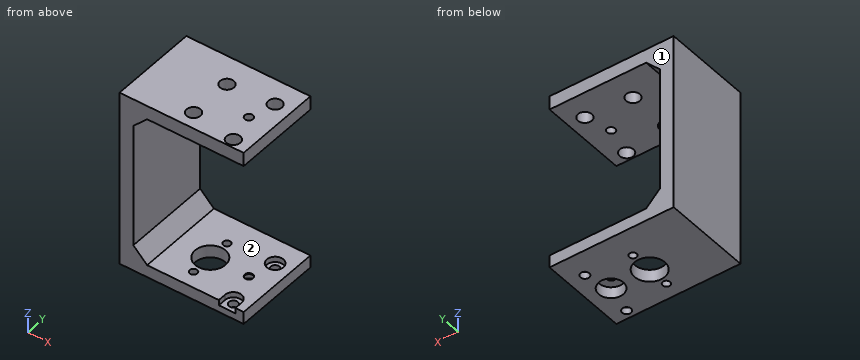
from build123d import *

# Parameters (mm, degrees)
SKETCH1_R           = 5.5
SKETCH1_R_2         = 4.45
BOSS_EXTRUDE1_DEPTH = 4.5
BOSS_EXTRUDE2_START = -0.4
SKETCH2_R           = 4.45
SKETCH2_R_2         = 1.5
BOSS_EXTRUDE2_DEPTH = 0.4
SKETCH3_R           = 1.6
CUT_EXTRUDE1_DEPTH  = 10
SKETCH4_R           = 1.35
CUT_EXTRUDE2_DEPTH  = 10
SKETCH5_W           = 45
SKETCH5_H           = 4.5
BOSS_EXTRUDE3_DEPTH = 4.5
SKETCH6_R           = 3
CUT_EXTRUDE4_DEPTH  = 2
SKETCH7_W           = 5
SKETCH7_H           = 32
BOSS_EXTRUDE4_DEPTH = 60
SKETCH8_W           = 5
SKETCH8_H           = 32
BOSS_EXTRUDE5_DEPTH = 40
CUT_EXTRUDE5_START  = -5
SKETCH11_R          = 2.5
SKETCH11_R_2        = 1.5
CUT_EXTRUDE5_DEPTH  = 5
CHAMFER1_SIZE       = 5


with BuildPart() as part:
    # Sketch1 → Boss-Extrude1 (new body)
    with BuildSketch(Plane.XY):
        Polygon((0, 27.5), (32.5, 27.5), (32.5, 0), (0, 0), (-12.5, 0), (-12.5, 27.5), align=None)
        with Locations((10, 13.75)):
            Circle(SKETCH1_R, mode=Mode.SUBTRACT)
        with Locations((24, 13.75)):
            Circle(SKETCH1_R_2, mode=Mode.SUBTRACT)
    extrude(amount=BOSS_EXTRUDE1_DEPTH)

    # Sketch2 → Boss-Extrude2 (add)
    with BuildSketch(Plane.XY.offset(4.5).offset(BOSS_EXTRUDE2_START)):
        with Locations((24, 13.75)):
            Circle(SKETCH2_R)
        with Locations((24, 13.75)):
            Circle(SKETCH2_R_2, mode=Mode.SUBTRACT)
    extrude(amount=BOSS_EXTRUDE2_DEPTH)

    # Sketch3 → Cut-Extrude1 (cut)
    with BuildSketch(Plane.XY.offset(4.5)):
        with Locations((26.5, 23)):
            Circle(SKETCH3_R)
        with Locations((26.5, 3)):
            Circle(SKETCH3_R)
    extrude(amount=-CUT_EXTRUDE1_DEPTH, mode=Mode.SUBTRACT)

    # Sketch4 → Cut-Extrude2 (cut)
    with BuildSketch(Plane.XY.offset(4.5)):
        with Locations((10, 21.75)):
            Circle(SKETCH4_R)
        with Locations((10, 5.75)):
            Circle(SKETCH4_R)
    extrude(amount=-CUT_EXTRUDE2_DEPTH, mode=Mode.SUBTRACT)

    # Sketch5 → Boss-Extrude3 (add)
    with BuildSketch(Plane.XY.offset(4.5)):
        with Locations((10, 29.75)):
            Rectangle(SKETCH5_W, SKETCH5_H)
    extrude(amount=-BOSS_EXTRUDE3_DEPTH)

    # Sketch6 → Cut-Extrude4 (cut)
    with BuildSketch(Plane.XY.offset(4.5)):
        with Locations((26.5, 23)):
            Circle(SKETCH6_R)
        with BuildLine():
            Line((23.5, 3), (23.5, 0))
            Line((23.5, 0), (29.5, 0))
            Line((29.5, 0), (29.5, 3))
            ThreePointArc((29.5, 3), (26.5, 6), (23.5, 3))
        make_face()
    extrude(amount=-CUT_EXTRUDE4_DEPTH, mode=Mode.SUBTRACT)

    # Sketch7 → Boss-Extrude4 (add)
    with BuildSketch(Plane.XY.offset(4.5)):
        with Locations((-10, 16)):
            Rectangle(SKETCH7_W, SKETCH7_H)
    extrude(amount=BOSS_EXTRUDE4_DEPTH)

    # Sketch8 → Boss-Extrude5 (add)
    with BuildSketch(Plane(origin=(-7.5, 0, 0), x_dir=(0, 0, -1), z_dir=(1, 0, 0))):
        with Locations((-62, 16)):
            Rectangle(SKETCH8_W, SKETCH8_H)
    extrude(amount=BOSS_EXTRUDE5_DEPTH)

    # Sketch11 → Cut-Extrude5 (cut)
    with BuildSketch(Plane.XY.offset(64.5).offset(CUT_EXTRUDE5_START)):
        with Locations((10, 21.75)):
            Circle(SKETCH11_R)
        with Locations((26.5, 23)):
            Circle(SKETCH11_R)
        with Locations((26.5, 3)):
            Circle(SKETCH11_R)
        with Locations((10, 5.75)):
            Circle(SKETCH11_R)
        with Locations((24, 13.75)):
            Circle(SKETCH11_R_2)
    extrude(amount=CUT_EXTRUDE5_DEPTH, mode=Mode.SUBTRACT)

    # Chamfer1
    chamfer1_edges = [part.edges().sort_by_distance(p)[0] for p in [
        (-7.5, 16, 59.5),
        (-7.5, 16, 4.5),
    ]]
    chamfer(chamfer1_edges, length=CHAMFER1_SIZE)


solid = part.part
Part model, mm, in its own coordinate system. Face numbers are marked on the shaded views. A direction names the side the tool comes from. Coordinates: 2 decimals unless noted, no trailing zeros. Order: outer loops, then holes, each group sorted by start corner. A loop starts at its lowest first (then second) coordinate and runs counter-clockwise, first axis right, second up.
(1) Tool access for the marked faces 1 and 2: list every direction of +Z, -Z, +X, -X, +Y, -Y with a clear straight run to the whole face (end or side of a thin tool).
Check sheet entries:
face 1: +Z, -Z, +X, -X, +Y
face 2: +X, +Y, -Y
(2) Probe L1, parallel to Y at x = 10, z = 3.5; L2, parallel to Y at x = 26.5, z = 61.1; L3, parallel to Z at x = 21, y = 25.5. List the from-to ranges inside material, lowest first.
Check sheet entries:
L1: y = 0 to 4.4, 7.1 to 8.25, 19.25 to 20.4, 23.1 to 32
L2: y = 0 to 0.5, 5.5 to 20.5, 25.5 to 32
L3: z = 0 to 4.5, 59.5 to 64.5
(3) Pin check, flat tips, straight feed: pin 1 Ø12 at (y, z) = (27, 32.5) entering from +X; pin 2 Ø1.8 at (x, y) = (27.5, 2.5) entering from +Z. Stop position of each tip, or through.
Check sheet entries:
pin 1: stops at x = -7.5
pin 2: stops at z = 2.5
(4) Slice it at D-D, the plane z = 55.5. Write the cut outline in (x, y).
Check sheet entries:
outline: (-12.5, 0) - (-6.5, 0) - (-6.5, 32) - (-12.5, 32) - close
(5) Slice it at C-C, the plane y = 10.5. Write the cut outline in (x, z), and give its area (3 significant figures).
Check sheet entries:
outline: (-12.5, 0) - (5.56, 0) - (5.56, 4.5) - (-2.5, 4.5) - (-7.5, 9.5) - (-7.5, 54.5) - (-2.5, 59.5) - (32.5, 59.5) - (32.5, 64.5) - (-12.5, 64.5) - close; (14.44, 0) - (20.96, 0) - (20.96, 4.1) - (27.04, 4.1) - (27.04, 0) - (32.5, 0) - (32.5, 4.5) - (14.44, 4.5) - close
area: 663 mm2
(6) Slice it at B-B, the plane y = 13.75. Write the cut outline in (x, z), and give its area (3 significant figures).
Check sheet entries:
outline: (-12.5, 0) - (4.5, 0) - (4.5, 4.5) - (-2.5, 4.5) - (-7.5, 9.5) - (-7.5, 54.5) - (-2.5, 59.5) - (22.5, 59.5) - (22.5, 64.5) - (-12.5, 64.5) - close; (15.5, 0) - (19.55, 0) - (19.55, 4.1) - (22.5, 4.1) - (22.5, 4.5) - (15.5, 4.5) - close; (25.5, 4.1) - (28.45, 4.1) - (28.45, 0) - (32.5, 0) - (32.5, 4.5) - (25.5, 4.5) - close; (25.5, 59.5) - (32.5, 59.5) - (32.5, 64.5) - (25.5, 64.5) - close
area: 625 mm2
(7) Slice it at A-A, the plane x = 10. Write the cut outline in (y, z), and give its area (3 significant figures).
Check sheet entries:
outline: (0, 0) - (4.4, 0) - (4.4, 4.5) - (0, 4.5) - close; (0, 59.5) - (3.25, 59.5) - (3.25, 64.5) - (0, 64.5) - close; (7.1, 0) - (8.25, 0) - (8.25, 4.5) - (7.1, 4.5) - close; (8.25, 59.5) - (19.25, 59.5) - (19.25, 64.5) - (8.25, 64.5) - close; (19.25, 0) - (20.4, 0) - (20.4, 4.5) - (19.25, 4.5) - close; (23.1, 0) - (32, 0) - (32, 4.5) - (23.1, 4.5) - close; (24.25, 59.5) - (32, 59.5) - (32, 64.5) - (24.25, 64.5) - close
area: 180 mm2
